Source: CAD feature listing. Evaluate the final solid. Frame: model axes, mm. Face numbers are marked on the shaded views. A direction names the side the tool comes from. Give positions to 0.01 mm unless a question says otherwise; leave off trailing zeros. Write each loop counter-clockwise with the first axis right and the second up, starting at its lowest first coordinate (ties: lowest second). Pieces come first, ordered by that corner, then holes. Notation, with made-up numbers: M -27,-26 L -2,-26 A13 ccw -2,-13 Z; hole C -20.75,-26.5 d11. An arc over 180 degrees is marked long. Answer as a JSON object with one key per item and string values. Group by question number.
```python
from build123d import *

# Parameters (mm, degrees)
F0_R     = 3.503318
F0_R_2   = 3.462973
F0_W     = 30.154734
F0_H     = 7.349356
F1_DEPTH = 25
F2_DEPTH = 25
F3_W     = 19
F3_H     = 27.151244
F4_DEPTH = 66.44531


with BuildPart() as f1:
    # F0 (on Front) → F1 (new body)
    with BuildSketch(Plane.XZ):
        with BuildLine():
            ThreePointArc((-30.65178, 6.35), (-37.00178, 0), (-30.65178, -6.35))
            Line((-30.65178, -6.35), (29.657688, -6.35))
            ThreePointArc((29.657688, -6.35), (36.007688, 0), (29.657688, 6.35))
            Line((29.657688, 6.35), (-0.497046, 6.35))
            Line((-0.497046, 6.35), (-30.65178, 6.35))
        make_face()
        with Locations((-30.65178, 0)):
            Circle(F0_R, mode=Mode.SUBTRACT)
        with Locations((29.657688, 0)):
            Circle(F0_R_2, mode=Mode.SUBTRACT)
        with Locations((14.580321, 10.024678)):
            Rectangle(F0_W, F0_H)
    extrude(amount=F1_DEPTH)

    # F0 (on Front) → F2 (join)
    with BuildSketch(Plane.XZ):
        with BuildLine():
            ThreePointArc((-30.65178, 6.35), (-37.00178, 0), (-30.65178, -6.35))
            Line((-30.65178, -6.35), (29.657688, -6.35))
            ThreePointArc((29.657688, -6.35), (36.007688, 0), (29.657688, 6.35))
            Line((29.657688, 6.35), (-0.497046, 6.35))
            Line((-0.497046, 6.35), (-30.65178, 6.35))
        make_face()
        with Locations((-30.65178, 0)):
            Circle(F0_R, mode=Mode.SUBTRACT)
        with Locations((29.657688, 0)):
            Circle(F0_R_2, mode=Mode.SUBTRACT)
        with Locations((14.580321, 10.024678)):
            Rectangle(F0_W, F0_H)
    extrude(amount=F2_DEPTH)

    # F3 (on Right) → F4 (cut, symmetric)
    with BuildSketch(Plane.YZ):
        with Locations((-12.5, -2.876266)):
            Rectangle(F3_W, F3_H)
    extrude(amount=F4_DEPTH, both=True, mode=Mode.SUBTRACT)


solid = f1.part
```
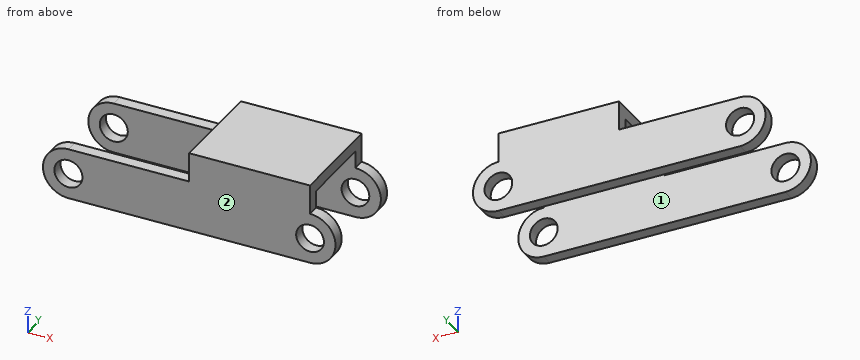
(1) Section A-A, the plane z = 9.75. Return loops of the section in (x, y).
(2) Section B-B, the plane x = -17.5. Return loops of the section in (y, z), plus the area to 3 significant figures.
(3) Section D-D, the plane x = 1. Return loops of the section in (y, z).
(4) Access query for the marked faces 1 and 2. Directions: +Z, -Z, +X, -X, +Y, -Y. A direction counts if a zero-diameter tool reaches every point of the face in a straight line with its end or side. Return the directions, or none.
(5) Ray query, L1, parallel to X at y = -24.1, z = 0; L2, parallel to Y at x = -4.5, z = 0; L3, parallel to Z at x = 19, y = -17.75. Return the intervals inside material, ascending. Write a range as [from, to].
(6) Section C-C, the plane z = 0. Return loops of the section in (x, y), plus the area to 3 significant figures.
(7) Contact query for flat-ended pins moving along their axis: pin 1 Ø3.5 at (x, y) = (-10.5, -1.5) entering from +Z; pin 2 Ø4 at (x, z) = (29.66, 0) entering from +Y; pin 3 Ø3.5 at (y, z) = (-8, 10.5) entering from -X; pin 4 Ø12 at (y, z) = (-19.5, 6.5) entering from +X. Output: stop coordinate, or through.
Reported:
{
 "1": {"outline": "M -0.5,-25 L 29.66,-25 L 29.66,-22 L -0.5,-22 Z; M -0.5,-3 L 29.66,-3 L 29.66,0 L -0.5,0 Z"},
 "2": {"outline": "M -25,-6.35 L -22,-6.35 L -22,6.35 L -25,6.35 Z; M -3,-6.35 L 0,-6.35 L 0,6.35 L -3,6.35 Z", "area": "76.2 mm2"},
 "3": {"outline": "M -25,-6.35 L -22,-6.35 L -22,10.7 L -3,10.7 L -3,-6.35 L 0,-6.35 L 0,13.7 L -25,13.7 Z"},
 "4": {"face 1": "-Z, +X, -X", "face 2": "+Z, -Z, +X, -X, -Y"},
 "5": {"L1": "x = [-37, -34.16], [-27.15, 26.19], [33.12, 36.01]", "L2": "y = [-25, -22], [-3, 0]", "L3": "z = [10.7, 13.7]"},
 "6": {"outline": "M -37,-25 L -34.16,-25 L -34.16,-22 L -37,-22 Z; M -37,-3 L -34.16,-3 L -34.16,0 L -37,0 Z; M -27.15,-25 L 26.19,-25 L 26.19,-22 L -27.15,-22 Z; M -27.15,-3 L 26.19,-3 L 26.19,0 L -27.15,0 Z; M 33.12,-25 L 36.01,-25 L 36.01,-22 L 33.12,-22 Z; M 33.12,-3 L 36.01,-3 L 36.01,0 L 33.12,0 Z", "area": "354 mm2"},
 "7": {"pin 1": "stops at z = 6.35", "pin 2": "passes through", "pin 3": "stops at x = -0.5", "pin 4": "stops at x = 35.92"}
}
